Design review of the part built by this model. Coordinates are the model's own, in mm. Face numbers are marked on the shaded views. Coordinates: 2 decimals unless noted, no trailing zeros. Loops run counter-clockwise (first coordinate to the right, second up) from the corner with the lowest first, then second, coordinate; pieces in that order, holes last. Notation, with made-up numbers: (-32, 83.5) -> (26, 83.5) arc R16 ccw to (26, 108.5) -> close; hole circle Ø10 at (24, -8). An arc over 180 degrees is marked (long way). Use a Markdown table: item, result. Add a question column.
Q1. Take a section at A-A on y = 29.5. Write out the cut boundary in (x, z), plus the area to 3 significant figures.
Q2. Take a section at D-D on y = 74.5. Write out the cut boundary in (x, z).
Q3. Take a section at B-B on z = -11.25. Write out the cut boundary in (x, y), plus the area to 3 significant figures.
Q4. Clearance check with flat-ended pins moving along their axes: pin 1 Ø9 at (x, z) = (-27, -13.5) entering from +Y; pin 2 Ø5 at (x, z) = (-42.05, -9.75) entering from -Y; pin 3 Ø1.2 at (x, y) = (-53, 77) entering from -Z; pin 4 Ø0.8 at (y, z) = (25, 0.5) entering from +X. State where each tip first meets the part, or that it passes through.
Q5. For probe 1 along X at (y, z) = (-27.85, -9.75); probe 2 along X at (y, z) = (-11.5, -7.5); probe 3 along Z at (x, y) = (-29, 82), list the stretches that pass through material, from the lowest coordinate up.
Q6. Take a section at C-C on x = -37. Write out the cut boundary in (y, z), plus the area to 3 significant figures.
Q7. Draft analysis for pull direction Z (two halves, no side actions). For the marked faces 1, 2 and 3, state which applies: pulls with the +Z half, pulls with the -Z half, needs draft (parallel to the pull), parting line crosses it, or undercut.
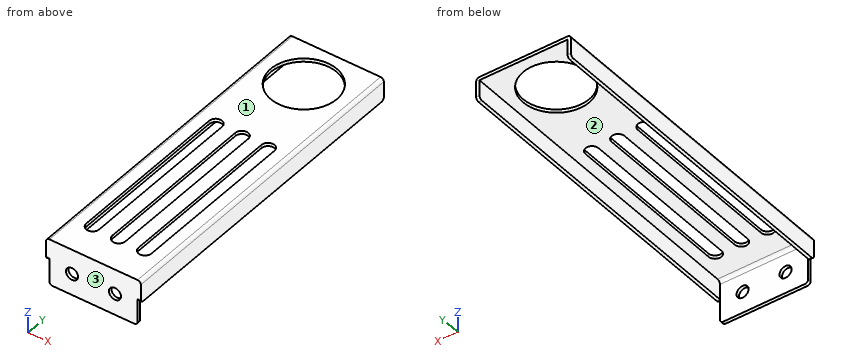
from build123d import *

# Parameters (mm, degrees)
CROQUIS1_W              = 40
CROQUIS1_H              = 148.5
SALIENTE_EXTRUIR1_DEPTH = 1.5
CROQUIS2_R              = 15
CORTAR_EXTRUIR1_DEPTH   = 1.5
CORTAR_EXTRUIR2_DEPTH   = 1.5
CROQUIS4_W              = 10
CROQUIS4_H              = 148.5
SALIENTE_EXTRUIR2_DEPTH = 1.5
CROQUIS5_W              = 10
CROQUIS5_H              = 148.5
SALIENTE_EXTRUIR3_DEPTH = 1.5
REDONDEO1_R             = 1.5
CROQUIS7_W              = 40
CROQUIS7_H              = 21
SALIENTE_EXTRUIR4_DEPTH = 1.5
REDONDEO2_R             = 1.5
CROQUIS8_R              = 2.75
CORTAR_EXTRUIR3_DEPTH   = 1.5
REDONDEO4_R             = 1.5


with BuildPart() as part:
    # Croquis1 → Saliente-Extruir1 (new body)
    with BuildSketch(Plane.XY):
        with Locations((-32.303310274, 45.797728257)):
            Rectangle(CROQUIS1_W, CROQUIS1_H)
    extrude(amount=SALIENTE_EXTRUIR1_DEPTH)

    # Croquis2 → Cortar-Extruir1 (cut)
    with BuildSketch(Plane.XY.offset(1.5)):
        with Locations((-32.303310274, 100.047728257)):
            Circle(CROQUIS2_R)
    extrude(amount=-CORTAR_EXTRUIR1_DEPTH, mode=Mode.SUBTRACT)

    # Croquis3 → Cortar-Extruir2 (cut)
    with BuildSketch(Plane.XY.offset(1.5)):
        with BuildLine():
            Line((-41.236643608, -12.952271743), (-41.236643608, 62.177728257))
            ThreePointArc((-41.236643608, 62.177728257), (-44.169976941, 65.11106159), (-47.103310274, 62.177728257))
            Line((-47.103310274, 62.177728257), (-47.103310274, -12.952271743))
            ThreePointArc((-47.103310274, -12.952271743), (-44.169976941, -15.885605076), (-41.236643608, -12.952271743))
        make_face()
        with BuildLine():
            Line((-29.369976941, -12.952271743), (-29.369976941, 62.177728257))
            ThreePointArc((-29.369976941, 62.177728257), (-32.303310274, 65.11106159), (-35.236643608, 62.177728257))
            Line((-35.236643608, 62.177728257), (-35.236643608, -12.952271743))
            ThreePointArc((-35.236643608, -12.952271743), (-32.303310274, -15.885605076), (-29.369976941, -12.952271743))
        make_face()
        with BuildLine():
            Line((-17.503310274, 62.177728257), (-17.503310274, -12.952271743))
            ThreePointArc((-17.503310274, -12.952271743), (-20.436643608, -15.885605076), (-23.369976941, -12.952271743))
            Line((-23.369976941, -12.952271743), (-23.369976941, 62.177728257))
            ThreePointArc((-23.369976941, 62.177728257), (-20.436643608, 65.11106159), (-17.503310274, 62.177728257))
        make_face()
    extrude(amount=-CORTAR_EXTRUIR2_DEPTH, mode=Mode.SUBTRACT)

    # Croquis4 → Saliente-Extruir2 (add)
    with BuildSketch(Plane.ZY.offset(52.303310274)):
        with Locations((-3.5, 45.797728257)):
            Rectangle(CROQUIS4_W, CROQUIS4_H)
    extrude(amount=SALIENTE_EXTRUIR2_DEPTH)

    # Croquis5 → Saliente-Extruir3 (add)
    with BuildSketch(Plane(origin=(-12.303310274, 0, 0), x_dir=(0, 0, -1), z_dir=(1, 0, 0))):
        with Locations((3.5, 45.797728257)):
            Rectangle(CROQUIS5_W, CROQUIS5_H)
    extrude(amount=SALIENTE_EXTRUIR3_DEPTH)

    # Redondeo1
    redondeo1_edges = [part.edges().sort_by_distance(p)[0] for p in [
        (-53.803310274, 45.797728257, 1.5),
        (-10.803310274, 45.797728257, 1.5),
    ]]
    fillet(redondeo1_edges, radius=REDONDEO1_R)

    # Croquis7 → Saliente-Extruir4 (add)
    with BuildSketch(Plane.XZ.offset(28.452271743)):
        with Locations((-32.303310274, -9)):
            Rectangle(CROQUIS7_W, CROQUIS7_H)
    extrude(amount=-SALIENTE_EXTRUIR4_DEPTH)

    # Redondeo2
    redondeo2_edges = [part.edges().sort_by_distance(p)[0] for p in [
        (-32.303310274, -26.952271743, 0),
    ]]
    fillet(redondeo2_edges, radius=REDONDEO2_R)

    # Croquis8 → Cortar-Extruir3 (cut)
    with BuildSketch(Plane(origin=(0, -28.452271743, 0), x_dir=(-1, 0, 0), z_dir=(0, -1, 0))):
        with Locations(Location((42.053310274, 9.75, 0), (0, 0, 90))):
            Circle(CROQUIS8_R)
        with Locations(Location((22.553310274, 9.75, 0), (0, 0, 90))):
            Circle(CROQUIS8_R)
    extrude(amount=-CORTAR_EXTRUIR3_DEPTH, mode=Mode.SUBTRACT)

    # Redondeo4
    redondeo4_edges = [part.edges().sort_by_distance(p)[0] for p in [
        (-52.303310274, -27.702271743, -19.5),
        (-12.303310274, -27.702271743, -19.5),
        (-53.053310274, -28.452271743, -8.5),
        (-53.053310274, 120.047728257, -8.5),
        (-11.553310274, -28.452271743, -8.5),
        (-11.553310274, 120.047728257, -8.5),
    ]]
    fillet(redondeo4_edges, radius=REDONDEO4_R)


solid = part.part
Answer list:
| question | item | result |
|---|---|---|
| 1 | outline | (-53.8, -8.5) -> (-52.3, -8.5) -> (-52.3, 0) -> (-47.1, 0) -> (-47.1, 1.5) -> (-52.3, 1.5) arc R1.5 ccw to (-53.8, 0) -> close; (-41.24, 0) -> (-35.24, 0) -> (-35.24, 1.5) -> (-41.24, 1.5) -> close; (-29.37, 0) -> (-23.37, 0) -> (-23.37, 1.5) -> (-29.37, 1.5) -> close; (-17.5, 0) -> (-12.3, 0) -> (-12.3, -8.5) -> (-10.8, -8.5) -> (-10.8, 0) arc R1.5 ccw to (-12.3, 1.5) -> (-17.5, 1.5) -> close |
| 1 | area | 62.6 mm² |
| 2 | outline | (-53.8, -8.5) -> (-52.3, -8.5) -> (-52.3, 0) -> (-12.3, 0) -> (-12.3, -8.5) -> (-10.8, -8.5) -> (-10.8, 0) arc R1.5 ccw to (-12.3, 1.5) -> (-52.3, 1.5) arc R1.5 ccw to (-53.8, 0) -> close |
| 3 | outline | (-52.3, -28.45) -> (-44.36, -28.45) -> (-44.36, -26.95) -> (-52.3, -26.95) -> close; (-39.75, -28.45) -> (-24.86, -28.45) -> (-24.86, -26.95) -> (-39.75, -26.95) -> close; (-20.25, -28.45) -> (-12.3, -28.45) -> (-12.3, -26.95) -> (-20.25, -26.95) -> close |
| 3 | area | 46.2 mm² |
| 4 | pin 1 | y = -26.95 |
| 4 | pin 2 | through |
| 4 | pin 3 | z = -8.5 |
| 4 | pin 4 | x = -10.81 |
| 5 | probe 1 | -52.3 to -44.8, -39.3 to -25.3, -19.8 to -12.3 |
| 5 | probe 2 | -53.8 to -52.3, -12.3 to -10.8 |
| 5 | probe 3 | 0 to 1.5 |
| 6 | outline | (-28.45, -19.5) -> (-26.95, -19.5) -> (-26.95, -1.5) arc R1.5 cw to (-25.45, 0) -> (85.8, 0) -> (85.8, 1.5) -> (-28.45, 1.5) -> close; (114.29, 0) -> (120.05, 0) -> (120.05, 1.5) -> (114.29, 1.5) -> close |
| 6 | area | 210 mm² |
| 7 | face 1 | pulls with the +Z half |
| 7 | face 2 | pulls with the -Z half |
| 7 | face 3 | needs draft |
